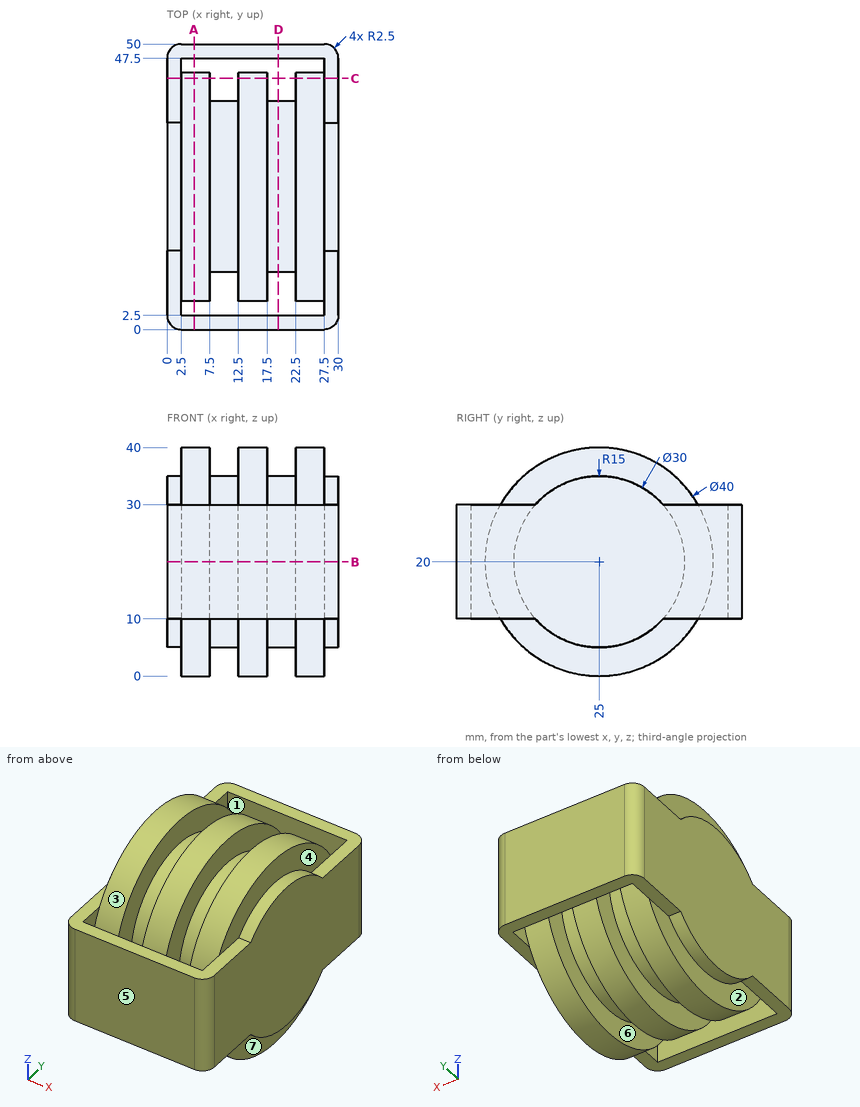
Geometry: see drawing. Coordinates: mm, zero at the bounding-box minimum. A direction names the side the tool comes from. Coordinates: 2 decimals unless noted, no trailing zeros. Order: outer loops, then holes, each group sorted by start corner. A loop starts at its lowest first (then second) coordinate and runs counter-clockwise, first axis right, second up. Notation, with made-up numbers: M 61.5,5 L 77.5,5 A25 ccw 77.5,26 Z; hole C -26.5,-4 d9. An arc over 180 degrees is marked long. Answer as CSV lines item,"result".
1. Pull-direction query (X, two-part tool) for the marked faces 5, 6 and 7; classes: released by +X, released by -X, zero draft, split by the parting line, or undercut.
Reported:
face 5,"zero draft"
face 6,"undercut"
face 7,"released by +X"
2. Section D-D (x = 19.5). Return the cut outline in (y, z), then the cut area to 3 significant figures.
Reported:
outline,"M 0,10 L 2.5,10 L 2.5,30 L 0,30 Z; C 25,20 d30; M 47.5,10 L 50,10 L 50,30 L 47.5,30 Z"
area,"807 mm2"
3. Access query for the marked faces 1, 2, 3 and 4. Directions: +Z, -Z, +X, -X, +Y, -Y. A direction counts if a zero-diameter tool reaches every point of the face in a straight line with its end or side. Return the directions, or none.
Reported:
face 1,"+Z, -Z"
face 2,"-Z, -X"
face 3,"none"
face 4,"+Z, +X"
4. Section C-C (y = 44). Return the cut outline in (x, z) (3 decimals).
Reported:
outline,"M 0,10 L 2.5,10 L 2.5,13.755 L 7.5,13.755 L 7.5,26.245 L 2.5,26.245 L 2.5,30 L 0,30 Z; M 12.5,13.755 L 17.5,13.755 L 17.5,26.245 L 12.5,26.245 Z; M 22.5,13.755 L 27.5,13.755 L 27.5,10 L 30,10 L 30,30 L 27.5,30 L 27.5,26.245 L 22.5,26.245 Z"
5. Section B-B (z = 20). State how many separate pieces and enclosed holes the cut face has, then the cut area to 3 significant figures.
Reported:
separate pieces,"1"
enclosed holes,"2"
area,"1,270 mm2"
6. Material intervals for line 1 (X direction, y = 9.5, z = 23); line 2 (X direction, y = 17, z = 33); line 3 (Y direction, x = 20, z = 17), sorted ascending. Write a range as from..to.
Reported:
line 1,"0..7.5, 12.5..17.5, 22.5..30"
line 2,"2.5..7.5, 12.5..17.5, 22.5..27.5"
line 3,"0..2.5, 10.3..39.7, 47.5..50"
7. Section A-A (x = 4.75). Return the cut outline in (y, z).
Reported:
outline,"M 0,10 L 2.5,10 L 2.5,30 L 0,30 Z; C 25,20 d40; M 47.5,10 L 50,10 L 50,30 L 47.5,30 Z"
8. First-contact query: P1, Ø6, axis at x = 14.5, y = 20, coming from the +Z side; P2, Ø4, axis at x = 21, y = 10.5, coming from the +Z side; P3, Ø12, axis at x = 14, y = 5.5, coming from the -Z side. Flat tips, straight axial feed; report the tip coordinate or a pass-through.
Reported:
P1,"z = 39.9"
P2,"z = 35.05"
P3,"z = 5.24"
